Work out the finished part from the listing and answer in its coordinate system (mm). A direction names the side the tool comes from. Coordinates: 2 decimals unless noted, no trailing zeros. One line per item, written item: value.
```python
from build123d import *
from build123d.topology import SkipClean

# Parameters (mm, degrees)
SKETCH1_R           = 45.85
SKETCH1_R_2         = 7.5
SKETCH1_R_3         = 2.1
BOSS_EXTRUDE1_DEPTH = 4
SKETCH1_6_R         = 1.48
SKETCH1_6_R_2       = 3
CUT_EXTRUDE1_DEPTH  = 2.22
BOSS_EXTRUDE2_START = 10.22
SKETCH1_7_R         = 45.85
SKETCH1_7_R_2       = 2.1
BOSS_EXTRUDE2_DEPTH = 10.22


with BuildPart() as part:
    # Sketch1 → Boss-Extrude1 (new body)
    with BuildSketch(Plane(origin=(0, 0, 0), x_dir=(1, 0, 0), z_dir=(0, 1, 0))):
        with Locations(Location((0, 0, 0), (0, 0, 270))):
            Circle(SKETCH1_R)
        with Locations(Location((0, 0, 0), (0, 0, 270))):
            Circle(SKETCH1_R_2, mode=Mode.SUBTRACT)
        with Locations(Location((-42.5, 0, 0), (0, 0, 270))):
            Circle(SKETCH1_R_3, mode=Mode.SUBTRACT)
        with Locations(Location((21.25, 36.806079661, 0), (0, 0, 270))):
            Circle(SKETCH1_R_3, mode=Mode.SUBTRACT)
        with Locations(Location((21.25, -36.806079661, 0), (0, 0, 270))):
            Circle(SKETCH1_R_3, mode=Mode.SUBTRACT)
    extrude(amount=-BOSS_EXTRUDE1_DEPTH)

    # Sketch1_6 → Cut-Extrude1 (cut)
    with BuildSketch(Plane(origin=(0, 0, 0), x_dir=(1, 0, 0), z_dir=(0, 1, 0))):
        with Locations(Location((-27.5, 0, 0), (0, 0, 270))):
            Circle(SKETCH1_6_R)
        with Locations(Location((-19.445436483, 19.445436483, 0), (0, 0, 270))):
            Circle(SKETCH1_6_R)
        with Locations(Location((0, 27.5, 0), (0, 0, 270))):
            Circle(SKETCH1_6_R)
        with Locations(Location((19.445436483, 19.445436483, 0), (0, 0, 270))):
            Circle(SKETCH1_6_R)
        with Locations(Location((27.5, 0, 0), (0, 0, 270))):
            Circle(SKETCH1_6_R)
        with Locations(Location((19.445436483, -19.445436483, 0), (0, 0, 270))):
            Circle(SKETCH1_6_R)
        with Locations(Location((0, -27.5, 0), (0, 0, 270))):
            Circle(SKETCH1_6_R)
        with Locations(Location((-19.445436483, -19.445436483, 0), (0, 0, 270))):
            Circle(SKETCH1_6_R)
        with Locations(Location((-36.680535028, 7.796688406, 0), (0, 0, 270))):
            Circle(SKETCH1_6_R_2)
        with Locations(Location((-36.680535028, -7.796688406, 0), (0, 0, 270))):
            Circle(SKETCH1_6_R_2)
        with Locations(Location((-30.338137289, 22.041946961, 0), (0, 0, 270))):
            Circle(SKETCH1_6_R_2)
        with Locations(Location((-30.338137289, -22.041946961, 0), (0, 0, 270))):
            Circle(SKETCH1_6_R_2)
        with Locations(Location((-18.75, -32.475952642, 0), (0, 0, 270))):
            Circle(SKETCH1_6_R_2)
        with Locations(Location((-3.919817373, -37.294571076, 0), (0, 0, 270))):
            Circle(SKETCH1_6_R_2)
        with Locations(Location((11.588137289, -35.664619361, 0), (0, 0, 270))):
            Circle(SKETCH1_6_R_2)
        with Locations(Location((25.092397738, -27.867930955, 0), (0, 0, 270))):
            Circle(SKETCH1_6_R_2)
        with Locations(Location((34.257954662, -15.252624115, 0), (0, 0, 270))):
            Circle(SKETCH1_6_R_2)
        with Locations(Location((37.5, 0, 0), (0, 0, 270))):
            Circle(SKETCH1_6_R_2)
        with Locations(Location((34.257954662, 15.252624115, 0), (0, 0, 270))):
            Circle(SKETCH1_6_R_2)
        with Locations(Location((25.092397738, 27.867930955, 0), (0, 0, 270))):
            Circle(SKETCH1_6_R_2)
        with Locations(Location((11.588137289, 35.664619361, 0), (0, 0, 270))):
            Circle(SKETCH1_6_R_2)
        with Locations(Location((-3.919817373, 37.294571076, 0), (0, 0, 270))):
            Circle(SKETCH1_6_R_2)
        with Locations(Location((-18.75, 32.475952642, 0), (0, 0, 270))):
            Circle(SKETCH1_6_R_2)
    extrude(amount=-CUT_EXTRUDE1_DEPTH, mode=Mode.SUBTRACT)

    # Sketch1_7 → Boss-Extrude2 (add)
    with SkipClean():  # the faces are left unmerged after this step: merging them gives an invalid solid
        with BuildSketch(Plane(origin=(0, 0, 0), x_dir=(1, 0, 0), z_dir=(0, 1, 0)).offset(BOSS_EXTRUDE2_START)):
            with Locations(Location((0, 0, 0), (0, 0, 270))):
                Circle(SKETCH1_7_R)
            with Locations(Location((-42.5, 0, 0), (0, 0, 270))):
                Circle(SKETCH1_7_R_2, mode=Mode.SUBTRACT)
            with Locations(Location((21.25, -36.806079661, 0), (0, 0, 270))):
                Circle(SKETCH1_7_R_2, mode=Mode.SUBTRACT)
            with BuildLine():
                ThreePointArc((36.883333333, 2.935936345), (39.39076704, 2.32916294), (40.5, 0))
                ThreePointArc((40.5, 0), (39.39076704, -2.32916294), (36.883333333, -2.935936345))
                ThreePointArc((36.883333333, -2.935936345), (36.191461227, -7.69273256), (34.888754523, -12.319691873))
                ThreePointArc((34.888754523, -12.319691873), (36.59166411, -13.367471546), (37.257954662, -15.252624115))
                ThreePointArc((37.257954662, -15.252624115), (35.6231437, -17.924001829), (32.500448736, -17.683914497))
                ThreePointArc((32.500448736, -17.683914497), (29.933628792, -21.748054335), (26.861593101, -25.445133446))
                ThreePointArc((26.861593101, -25.445133446), (27.767055295, -26.50917897), (28.092397738, -27.867930955))
                ThreePointArc((28.092397738, -27.867930955), (25.872343464, -30.764771418), (22.497941295, -29.37418318))
                ThreePointArc((22.497941295, -29.37418318), (18.5, -32.04293994), (14.189818202, -34.170880284))
                ThreePointArc((14.189818202, -34.170880284), (14.486847583, -34.891651942), (14.588137289, -35.664619361))
                ThreePointArc((14.588137289, -35.664619361), (11.748752331, -38.660316744), (8.605335417, -35.985388734))
                ThreePointArc((8.605335417, -35.985388734), (3.867553141, -36.797310129), (-0.935505175, -36.988171489))
                ThreePointArc((-0.935505175, -36.988171489), (-0.92374189, -37.141170608), (-0.919817373, -37.294571076))
                ThreePointArc((-0.919817373, -37.294571076), (-4.385552663, -40.258199029), (-6.775211132, -36.37439366))
                ThreePointArc((-6.775211132, -36.37439366), (-11.433628792, -35.189091103), (-15.899071208, -33.409871815))
                ThreePointArc((-15.899071208, -33.409871815), (-20.25, -35.074028853), (-20.984262125, -30.47393547))
                ThreePointArc((-20.984262125, -30.47393547), (-24.757832435, -27.496358543), (-28.113543391, -24.054701786))
                ThreePointArc((-28.113543391, -24.054701786), (-32.765188272, -23.805302718), (-31.564943561, -19.304256991))
                ThreePointArc((-31.564943561, -19.304256991), (-33.801181933, -15.049255794), (-35.466928517, -10.540255288))
                ThreePointArc((-35.466928517, -10.540255288), (-39.61497783, -8.420423478), (-36.687759497, -4.796697105))
                ThreePointArc((-36.687759497, -4.796697105), (-37, 0), (-36.687759497, 4.796697105))
                ThreePointArc((-36.687759497, 4.796697105), (-39.61497783, 8.420423478), (-35.466928517, 10.540255288))
                ThreePointArc((-35.466928517, 10.540255288), (-33.801181933, 15.049255794), (-31.564943561, 19.304256991))
                ThreePointArc((-31.564943561, 19.304256991), (-32.765188272, 23.805302718), (-28.113543391, 24.054701786))
                ThreePointArc((-28.113543391, 24.054701786), (-24.757832435, 27.496358543), (-20.984262125, 30.47393547))
                ThreePointArc((-20.984262125, 30.47393547), (-20.25, 35.074028853), (-15.899071208, 33.409871815))
                ThreePointArc((-15.899071208, 33.409871815), (-11.433628792, 35.189091103), (-6.775211132, 36.37439366))
                ThreePointArc((-6.775211132, 36.37439366), (-4.385552663, 40.258199029), (-0.919817373, 37.294571076))
                ThreePointArc((-0.919817373, 37.294571076), (-0.92374189, 37.141170608), (-0.935505175, 36.988171489))
                ThreePointArc((-0.935505175, 36.988171489), (3.867553141, 36.797310129), (8.605335417, 35.985388734))
                ThreePointArc((8.605335417, 35.985388734), (11.748752331, 38.660316744), (14.588137289, 35.664619361))
                ThreePointArc((14.588137289, 35.664619361), (14.486847583, 34.891651942), (14.189818202, 34.170880284))
                ThreePointArc((14.189818202, 34.170880284), (18.5, 32.04293994), (22.497941295, 29.37418318))
                ThreePointArc((22.497941295, 29.37418318), (25.872343464, 30.764771418), (28.092397738, 27.867930955))
                ThreePointArc((28.092397738, 27.867930955), (27.767055295, 26.50917897), (26.861593101, 25.445133446))
                ThreePointArc((26.861593101, 25.445133446), (29.933628792, 21.748054335), (32.500448736, 17.683914497))
                ThreePointArc((32.500448736, 17.683914497), (35.6231437, 17.924001829), (37.257954662, 15.252624115))
                ThreePointArc((37.257954662, 15.252624115), (36.59166411, 13.367471546), (34.888754523, 12.319691873))
                ThreePointArc((34.888754523, 12.319691873), (36.191461227, 7.69273256), (36.883333333, 2.935936345))
            make_face(mode=Mode.SUBTRACT)
            with Locations(Location((21.25, 36.806079661, 0), (0, 0, 270))):
                Circle(SKETCH1_7_R_2, mode=Mode.SUBTRACT)
        extrude(amount=-BOSS_EXTRUDE2_DEPTH)


solid = part.part
```
Item 1: Section A-A, the plane y = 1.25 is taken. Give the number of separate pieces and of enclosed holes in the cut face, then the cut area to 3 significant figures.
Evaluation:
separate pieces: 1
enclosed holes: 4
area: 2,000 mm2
Item 2: Consider probe 1 along X at (y, z) = (-1, 0); probe 2 along X at (y, z) = (-1.25, -20); probe 3 along X at (y, z) = (-0.95, -27.5). Determine where each line is inside the solid, lowest interval first.
Evaluation:
probe 1: x = -45.85 to -44.6, -40.4 to -28.98, -26.02 to -7.5, 7.5 to 26.02, 28.98 to 34.5, 40.5 to 45.85
probe 2: x = -41.26 to -32.54, -28.14 to -20.82, -18.07 to 18.07, 20.82 to 41.26
probe 3: x = -36.69 to -1.48, 1.48 to 22.12, 28.07 to 36.69
Item 3: Which of the six approach directions +Z, -Z, +X, -X, +Y, -Y give full straight-line access (tool end or side, diameter ignored) to faces 3 (the face through (23.332, 3.21, -37.079)), 4 (the face through (-4, -2.22, -37))?
Evaluation:
face 3: +Y, -Y
face 4: +Y
Item 4: Given pin 1 (3 mm diameter, centred on y = 7, z = -8, fed in from -X); pin 2 (4.5 mm diameter, centred on x = 19.45, z = -19.45, fed in from +Y); pin 3 (2.5 mm diameter, centred on x = 0, z = -27.5, fed in from +Y), each flat-ended and moving along its own axis, determine where each tip first touches the part or whether it passes through.
Evaluation:
pin 1: stops at x = -45.39
pin 2: stops at y = 0
pin 3: stops at y = -2.22
Item 5: Determine the mould class of faces 1 (the face through (25, -2.22, -28)), 2 (the face through (45.46, 3.21, -5.97)) for opening direction Z: +Z half, -Z half, draft (parallel to the pull), parting line (faces both ways), or undercut.
Evaluation:
face 1: undercut
face 2: parting line
